```python
from build123d import *

# Parameters (mm, degrees)
F1_DEPTH = 25.4
F2_R     = 2.2606
F3_DEPTH = 3.175
F4_R     = 2.2606
F5_DEPTH = 3.175
F6_W     = 6.35
F6_H     = 25.4
F7_DEPTH = 3.175


with BuildPart() as f1:
    # F0 (on Right) → F1 (new body, symmetric)
    with BuildSketch(Plane.YZ):
        Polygon((0, 31.75), (0, 0), (-31.75, 0), (-31.75, -3.175), (0, -3.175), (0, -57.15), (80.690128, -57.15), (108.560832, -29.279296), (106.315768, -27.034232), (79.375, -53.975), (3.175, -53.975), (3.175, 31.75), align=None)
    extrude(amount=F1_DEPTH, both=True)

    # F2 (on face) → F3 (cut, through all)
    with BuildSketch(Plane(origin=(0, 3.175, 0), x_dir=(-1, 0, 0), z_dir=(0, 1, 0))):
        with Locations((15.875, 15.875)):
            Circle(F2_R)
        with Locations((-15.875, 15.875)):
            Circle(F2_R)
    extrude(amount=-F3_DEPTH, mode=Mode.SUBTRACT)

    # F4 (on face) → F5 (cut, through all)
    with BuildSketch(Plane.XY):
        with Locations((15.875, -15.875)):
            Circle(F4_R)
        with Locations((-15.875, -15.875)):
            Circle(F4_R)
    extrude(amount=-F5_DEPTH, mode=Mode.SUBTRACT)

    # F6 (on face) → F7 (cut, through all)
    with BuildSketch(Plane(origin=(0, 68.920064, -68.920064), x_dir=(-1, 0, 0), z_dir=(0, 0.707107, -0.707107))):
        with BuildLine():
            ThreePointArc((-12.7, 48.368529), (-15.875, 51.543529), (-19.05, 48.368529))
            Line((-19.05, 48.368529), (-12.7, 48.368529))
        make_face()
        with Locations((-15.875, 35.668529)):
            Rectangle(F6_W, F6_H)
        with BuildLine():
            Line((-12.7, 22.968529), (-19.05, 22.968529))
            ThreePointArc((-19.05, 22.968529), (-15.875, 19.793529), (-12.7, 22.968529))
        make_face()
        with BuildLine():
            ThreePointArc((19.05, 48.368529), (15.875, 51.543529), (12.7, 48.368529))
            Line((12.7, 48.368529), (19.05, 48.368529))
        make_face()
        with Locations((15.875, 35.668529)):
            Rectangle(F6_W, F6_H)
        with BuildLine():
            Line((19.05, 22.968529), (12.7, 22.968529))
            ThreePointArc((12.7, 22.968529), (15.875, 19.793529), (19.05, 22.968529))
        make_face()
    extrude(amount=-F7_DEPTH, mode=Mode.SUBTRACT)


solid = f1.part
```
CAD build for the part. Positions are in the model's coordinates, mm. A direction names the side the tool comes from. Round coordinates to 2 decimals unless told otherwise and drop trailing zeros. Write each loop counter-clockwise with the first axis right and the second up, starting at its lowest first coordinate (ties: lowest second). Pieces come first, ordered by that corner, then holes. Notation, with made-up numbers: (88, 58.5) - (102, 58.5) arc R11 cw to (102, 64.5) - close; hole circle Ø8 at (-23, 87). An arc over 180 degrees is marked (long way). Write item = value, one per line. Start each with the question number.
Q1. Band-saw the part on C-C (y = 97.5). Give the cut face in (x, z).
Q2. Drop flat-ended pins along their axis: pin 1 (1.5 mm diameter, centred on x = -1, z = -36.5, fed in from -Y); pin 2 (3.5 mm diameter, centred on x = -15.875, y = -15.875, fed in from +Z); pin 3 (5 mm diameter, centred on x = -5, y = 24.5, fed in from +Z) (3 decimals); pin 4 (9.5 mm diameter, centred on x = 12, y = -11, fed in from +Z). Give the stop position or say it passes through.
Q3. Mould opens along Y. For faces 5 (the flat face through (0, 0, -30)), 6 (the flat face through (0, 3.175, -12)), 7 (the flat face through (-25.4, 2, -26)) say: pulls with the +Y half, pulls with the -Y half, needs draft (parallel to the pull), parting line crosses it, or undercut.
Q4. Band-saw the part on A-A (z = -46). Give the cut face in (x, y) (3 decimals), then the cut area to 3 significant figures.
Q5. Band-saw the part on D-D (z = -16). Give the cut face in (x, y) (3 decimals).
Q6. Band-saw the part on B-B (x = -21.5). Give the cut face in (y, z) (3 decimals), then the cut area to 3 significant figures.
Q7. Probe L1, parallel to Y at x = 8.5, z = 14.5 (3 decimals); L2, parallel to Z at x = -10, y = 11 (3 decimals); L3, parallel to Y at x = -23, z = -29 (3 decimals). List the from-to ranges inside material, lowest first. Write a range as from..to.
Q8. Which spindle directions (+Z, -Z, +X, -X, +Y, -Y) get a long thin tool onto all of the face, cutting with end or side? Do faces 1 (the cylindrical face through (15.81, 104.26, -31.37)), 2 (the flat face through (0, 42, -53.975)), 3 (the flat face through (0, 0, 16)), 4 (the flat face through (0, -16, -3.175)). Say none if no direction does.
Answers below:
q1.outline = (-25.4, -40.34) - (-19.05, -40.34) - (-19.05, -35.85) - (-25.4, -35.85) - close; (-12.7, -40.34) - (12.7, -40.34) - (12.7, -35.85) - (-12.7, -35.85) - close; (19.05, -40.34) - (25.4, -40.34) - (25.4, -35.85) - (19.05, -35.85) - close
q2.pin_1 = 0
q2.pin_2 = through
q2.pin_3 = -53.975
q2.pin_4 = 0
q3.face_5 = pulls with the -Y half
q3.face_6 = undercut
q3.face_7 = needs draft
q4.outline = (-25.4, 0) - (25.4, 0) - (25.4, 3.175) - (-25.4, 3.175) - close; (-25.4, 87.35) - (-19.05, 87.35) - (-19.05, 91.84) - (-25.4, 91.84) - close; (-12.7, 87.35) - (12.7, 87.35) - (12.7, 91.84) - (-12.7, 91.84) - close; (19.05, 87.35) - (25.4, 87.35) - (25.4, 91.84) - (19.05, 91.84) - close
q4.area = 332 mm2
q5.outline = (-25.4, 0) - (25.4, 0) - (25.4, 3.175) - (-25.4, 3.175) - close
q6.outline = (-31.75, -3.175) - (0, -3.175) - (0, -57.15) - (80.69, -57.15) - (108.561, -29.279) - (106.316, -27.034) - (79.375, -53.975) - (3.175, -53.975) - (3.175, 31.75) - (0, 31.75) - (0, 0) - (-31.75, 0) - close
q6.area = 750 mm2
q7.L1 = 0..3.175
q7.L2 = -57.15..-53.975
q7.L3 = 0..3.175, 104.35..108.282
q8.face_1 = -Z
q8.face_2 = +Z, +X, -X
q8.face_3 = +Z, +X, -X, -Y
q8.face_4 = -Z, +X, -X, -Y
